Could you check a few things on this model? Use its own coordinates, in mm. A direction names the side the tool comes from. Give positions to 0.01 mm unless a question says otherwise; leave off trailing zeros. Write each loop counter-clockwise with the first axis right and the second up, starting at its lowest first coordinate (ties: lowest second). Pieces come first, ordered by that corner, then holes. Notation, with made-up numbers: M 77,7.5 L 126,7.5 A19 ccw 126,18.5 Z; hole C -39.5,74.25 d7. An arc over 180 degrees is marked long. Use one line per item in the form item = value.
from build123d import *

# Parameters (mm, degrees)
SKETCH1_R           = 15
BOSS_EXTRUDE1_DEPTH = 10
SKETCH2_W           = 15
SKETCH2_H           = 15
CUT_EXTRUDE1_DEPTH  = 3
SKETCH3_R           = 4.7625
CUT_EXTRUDE2_DEPTH  = 4.7625


with BuildPart() as part:
    # Sketch1 → Boss-Extrude1 (new body)
    with BuildSketch(Plane(origin=(0, 0, 0), x_dir=(0, 0, -1), z_dir=(1, 0, 0))):
        Circle(SKETCH1_R)
    extrude(amount=BOSS_EXTRUDE1_DEPTH)

    # Sketch2 → Cut-Extrude1 (cut)
    with BuildSketch(Plane.ZY):
        Rectangle(SKETCH2_W, SKETCH2_H)
    extrude(amount=-CUT_EXTRUDE1_DEPTH, mode=Mode.SUBTRACT)

    # Sketch3 → Cut-Extrude2 (cut)
    with BuildSketch(Plane(origin=(10, 0, 0), x_dir=(0, 0, -1), z_dir=(1, 0, 0))):
        Circle(SKETCH3_R)
    extrude(amount=-CUT_EXTRUDE2_DEPTH, mode=Mode.SUBTRACT)

    # Sketch4 → Cut-Revolve1 (revolve, cut)
    with BuildSketch(Plane.XY):
        Polygon((5.2375, 4.7625), (3, 1.25), (3, 0), (5.2375, 0), align=None)
    revolve(axis=Axis((5.2375, 0, 0), (1, 0, 0)), mode=Mode.SUBTRACT)


solid = part.part
1) I want a section at C-C, the plane x = 2.5. Please give me the cut outline in (y, z), plus the area to 3 significant figures.
Checked values:
outline = C 0,0 d30; hole M -7.5,-7.5 L 7.5,-7.5 L 7.5,7.5 L -7.5,7.5 Z
area = 482 mm2
2) For pin 1 Ø6 at (x, z) = (3.5, -4.5) entering from -Y; pin 2 Ø2.5 at (x, y) = (1, 1.5) entering from -Z; pin 3 Ø1 at (x, z) = (3, 2) entering from +Y, each with a flat end and sliding along its axis, tell me the tip position at first contact or that it passes through.
Checked values:
pin_1 = -14.92
pin_2 = -15
pin_3 = 14.92
3) For faces 5 (the flat face through (1, 0, 7.5)), 6 (the cylindrical face through (7.65, -2.9, 3.78)), 7 (the flat face through (10, 4, 4)), which set-ups out of +Z, -Z, +X, -X, +Y, -Y let a thin tool reach every point of the face, with its end or its side?
Checked values:
face_5 = -X
face_6 = +X
face_7 = +Z, -Z, +X, +Y, -Y
4) I want a section at D-D, the plane y = 6.5. Please give me the cut outline in (x, z), plus the area to 3 significant figures.
Checked values:
outline = M 0,-13.52 L 10,-13.52 L 10,13.52 L 0,13.52 L 0,7.5 L 3,7.5 L 3,-7.5 L 0,-7.5 Z
area = 225 mm2
5) Thinking about a two-plate mould opening in Y: for faces 1 (the flat face through (0, -10, 0)), 2 (the flat face through (1, 7.5, 0)), 3 (the cylindrical face through (4.93, 0.66, 14.985)), 4 (the flat face through (3, 0, -2)), which applies, released by +Y, released by -Y, zero draft, split by the parting line, or undercut?
Checked values:
face_1 = zero draft
face_2 = undercut
face_3 = split by the parting line
face_4 = undercut
6) If I drill on L1, parallel to Y at x = 6.9, z = 0; L2, parallel to X at y = -5.5, z = -4; L3, parallel to Y at x = 1, z = 4, over which ranges is the centre line in solid material (lowest first)?
Checked values:
L1 = -15 to -4.76, 4.76 to 15
L2 = 3 to 10
L3 = -14.46 to -7.5, 7.5 to 14.46
7) I want a section at A-A, the plane y = 0. Please give me the cut outline in (x, z), plus the area to 3 significant figures.
Checked values:
outline = M 0,-15 L 10,-15 L 10,-4.76 L 5.24,-4.76 L 3,-1.25 L 3,-7.5 L 0,-7.5 Z; M 0,7.5 L 3,7.5 L 3,1.25 L 5.24,4.76 L 10,4.76 L 10,15 L 0,15 Z
area = 196 mm2
